Build history of the part. All positions in model axes, mm. Round coordinates to 2 decimals unless told otherwise and drop trailing zeros. Order: outer loops, then holes, each group sorted by start corner. A loop starts at its lowest first (then second) coordinate and runs counter-clockwise, first axis right, second up. Notation, with made-up numbers: (8, 24) -> (14, 24) arc R10 ccw to (14, 30) -> close; hole circle Ø4 at (27, -36). An arc over 180 degrees is marked (long way). Write item = value, one per line.
from build123d import *

# Parameters (mm, degrees)
SKETCH1_R           = 2.4892
BOSS_EXTRUDE1_DEPTH = 6.35
FILLET1_R           = 6.35


with BuildPart() as part:
    # Sketch1 → Boss-Extrude1 (new body)
    with BuildSketch(Plane.XY):
        Polygon((0, 0), (0, 127), (25.4, 127), (127, 25.4), (127, 0), align=None)
        with Locations((12.7, 12.7)):
            Circle(SKETCH1_R, mode=Mode.SUBTRACT)
        with Locations((38.1, 12.7)):
            Circle(SKETCH1_R, mode=Mode.SUBTRACT)
        with Locations((63.5, 12.7)):
            Circle(SKETCH1_R, mode=Mode.SUBTRACT)
        with Locations((12.7, 38.1)):
            Circle(SKETCH1_R, mode=Mode.SUBTRACT)
        with Locations((12.7, 63.5)):
            Circle(SKETCH1_R, mode=Mode.SUBTRACT)
        with Locations((12.7, 88.9)):
            Circle(SKETCH1_R, mode=Mode.SUBTRACT)
        with Locations((12.7, 114.3)):
            Circle(SKETCH1_R, mode=Mode.SUBTRACT)
        with Locations((88.9, 12.7)):
            Circle(SKETCH1_R, mode=Mode.SUBTRACT)
        with Locations((114.3, 12.7)):
            Circle(SKETCH1_R, mode=Mode.SUBTRACT)
    extrude(amount=BOSS_EXTRUDE1_DEPTH)

    # Fillet1
    fillet1_edges = [part.edges().sort_by_distance(p)[0] for p in [
        (127, 0, 3.175),
        (0, 0, 3.175),
        (0, 127, 3.175),
        (25.4, 127, 3.175),
        (127, 25.4, 3.175),
    ]]
    fillet(fillet1_edges, radius=FILLET1_R)


solid = part.part
Q1. Cut at A-A, the plane y = 12.7. List the corners of the cut face in (x, z), and give its area (3 significant figures).
Check values:
outline = (0, 0) -> (10.21, 0) -> (10.21, 6.35) -> (0, 6.35) -> close; (15.19, 0) -> (35.61, 0) -> (35.61, 6.35) -> (15.19, 6.35) -> close; (40.59, 0) -> (61.01, 0) -> (61.01, 6.35) -> (40.59, 6.35) -> close; (65.99, 0) -> (86.41, 0) -> (86.41, 6.35) -> (65.99, 6.35) -> close; (91.39, 0) -> (111.81, 0) -> (111.81, 6.35) -> (91.39, 6.35) -> close; (116.79, 0) -> (127, 0) -> (127, 6.35) -> (116.79, 6.35) -> close
area = 648 mm²
Q2. Cut at D-D, the plane x = 114.3. List the corners of the cut face in (y, z), and give its area (3 significant figures).
Check values:
outline = (0, 0) -> (10.21, 0) -> (10.21, 6.35) -> (0, 6.35) -> close; (15.19, 0) -> (38.1, 0) -> (38.1, 6.35) -> (15.19, 6.35) -> close
area = 210 mm²
Q3. Mould opens along Y. For faces 1 (the face through (1.81, 125.09, 3.22)), 2 (the face through (12.16, 111.87, 3.13)), 3 (the face through (50, 50, 0)), 4 (the face through (111.813, 12.809, 3.131)) say: released by +Y, released by -Y, zero draft, split by the parting line, or undercut.
Check values:
face_1 = released by +Y
face_2 = undercut
face_3 = zero draft
face_4 = undercut
Q4. Probe probe 1 along Y at (x, z) = (12.7, 5); probe 2 along X at (y, z) = (113.5, 4.5); probe 3 along Y at (x, z) = (113, 2.75). List the from-to ranges inside material, lowest first.
Check values:
probe_1 = 0 to 10.21, 15.19 to 35.61, 40.59 to 61.01, 65.99 to 86.41, 91.39 to 111.81, 116.79 to 127
probe_2 = 0 to 10.34, 15.06 to 38.9
probe_3 = 0 to 10.58, 14.82 to 39.4
Q5. Cut at C-C, the plane y = 88.9. List the corners of the cut face in (x, z).
Check values:
outline = (0, 0) -> (10.21, 0) -> (10.21, 6.35) -> (0, 6.35) -> close; (15.19, 0) -> (63.5, 0) -> (63.5, 6.35) -> (15.19, 6.35) -> close
Q6. Flat gauge pin, fed straight in: pin 1 (4 mm diameter, centred on x = 12.7, y = 38.1, fed in from +Z). Where does the tip first touch, or does it go through?
Check values:
pin_1 = through
